Read the model definition and answer for the solid it produces. Units are mm, in the model's axes. A direction names the side the tool comes from. Coordinates: 2 decimals unless noted, no trailing zeros. Order: outer loops, then holes, each group sorted by start corner. A loop starts at its lowest first (then second) coordinate and runs counter-clockwise, first axis right, second up. Notation, with made-up numbers: (53.25, -6) - (101.25, -6) arc R14 cw to (101.25, 16) - close; hole circle Ø2 at (27.5, 9). An arc over 180 degrees is marked (long way). Use one line per item in the form item = value. Start each with the question number.
Autodesk Inventor part; units mm, degrees
ref_plane "YZ Plane" through (0, 0, 0) normal (1, 0, 0) x (0, 1, 0)
ref_plane "XZ Plane" through (0, 0, 0) normal (0, 1, 0) x (-1, 0, 0)
ref_plane "XY Plane" through (0, 0, 0) normal (0, 0, 1) x (1, 0, 0)
sketch "Sketch1" plane through (0, 0, 0) normal (0, 0, 1) x (1, 0, 0)
  circle A0 centre (0, 0) radius 38.1824
extrude "Extrusion1" add sketch "Sketch1" along normal blind 50.8
sketch "Sketch2" plane through (0, 0, 0) normal (0, 0, -1) x (-1, 0, 0)
  line L0 (-10.125, -10.125) -> (10.125, -10.125)
  line L1 (-10.125, 10.125) -> (-10.125, -10.125)
  line L2 (10.125, 10.125) -> (-10.125, 10.125)
  line L3 (10.125, -10.125) -> (10.125, 10.125)
  circle A0 centre (0, 0) radius 25.4
  circle A1 centre (0, 0) radius 25.5
  dimension "d22" = 51
  dimension "d23" = 50.8
extrude "Extrusion2" cut sketch "Sketch2" against normal blind 5 contours L1 L2 L3 L0 | A0 | A1
sketch "Sketch4" plane through (0, 0, 50.8) normal (0, 0, 1) x (1, 0, 0)
  circle A0 centre (0, 0) radius 25.5
  circle A1 centre (0, 0) radius 25.5
extrude "Extrusion4" cut sketch "Sketch4" against normal blind 44.45
ref_plane "Work Plane1" through (0, 10, -2.54) normal (1, 0, 0) x (0, -1, 0)
sketch "Sketch5" plane through (0, 10, -2.54) normal (1, 0, 0) x (0, -1, 0)
  line L0 (-28.1824, -53.34) -> (48.1824, -53.34)
  ellipse E0 centre (10, -53.34) end of major axis (28.5443, -53.34) minor radius 32.3873 (28.5443, -53.34) -> (-8.5443, -53.34) ccw
  point P0 (10, -2.54)
extrude "Extrusion5" cut sketch "Sketch5" along normal through all both and the other way through all
sketch "Sketch6" plane through (0, 10, -2.54) normal (1, 0, 0) x (0, -1, 0)
  point P0 (10, -2.54)
sketch "Sketch7" plane through (0, 0, 6.35) normal (0, 0, 1) x (1, 0, 0)
  circle A0 centre (0, 0) radius 3.975
  circle A1 centre (0, 0) radius 4.1
  dimension "d12" = 8.2
extrude "Extrusion6" cut sketch "Sketch7" against normal blind 10 contours A0 | A1
sketch "Sketch8" plane through (0, 0, 0) normal (0, 0, -1) x (-1, 0, 0)
  circle A0 centre (0, 0) radius 25.4
  line L0 (-17.5031, 18.5443) -> (-33.3767, 18.5443)
  line L1 (-33.3767, -18.5443) -> (-17.5031, -18.5443)
  line L2 (17.5031, -18.5443) -> (33.3767, -18.5443)
  line L3 (33.3767, 18.5443) -> (17.5031, 18.5443)
  circle A1 centre (0, 31.8008) radius 3.4055
  circle A2 centre (-15.9004, 27.5403) radius 3.4055
  circle A3 centre (-27.5403, 15.9004) radius 3.4055
  circle A4 centre (-31.8008, 0) radius 3.4055
  circle A5 centre (-27.5403, -15.9004) radius 3.4055
  circle A6 centre (-15.9004, -27.5403) radius 3.4055
  circle A7 centre (0, -31.8008) radius 3.4055
  circle A8 centre (15.9004, -27.5403) radius 3.4055
  circle A9 centre (27.5403, -15.9004) radius 3.4055
  circle A10 centre (31.8008, 0) radius 3.4055
  circle A11 centre (27.5403, 15.9004) radius 3.4055
  circle A12 centre (15.9004, 27.5403) radius 3.4055
  dimension "d15" = 6.811
  dimension "d18" = 360
sketch "Sketch9" plane through (0, 0, 0) normal (0, 0, -1) x (-1, 0, 0)
  circle A0 centre (0, 31.8008) radius 3.4055
  circle A1 centre (15.9004, 27.5403) radius 3.4055
  circle A2 centre (-15.9004, 27.5403) radius 3.4055
  circle A3 centre (-15.9004, -27.5403) radius 3.4055
  circle A4 centre (0, -31.8008) radius 3.4055
  circle A5 centre (15.9004, -27.5403) radius 3.4055
  circle A6 centre (0, 31.8008) radius 3.4055
  circle A7 centre (15.9004, 27.5403) radius 3.4055
  circle A8 centre (-15.9004, 27.5403) radius 3.4055
  circle A9 centre (-15.9004, -27.5403) radius 3.4055
  circle A10 centre (0, -31.8008) radius 3.4055
  circle A11 centre (15.9004, -27.5403) radius 3.4055
  point P0 (0, 0)
extrude "Extrusion7" cut sketch "Sketch8" against normal blind 48 contours A1 | A2 | A6 | A7 | A8 | A12
properties part number "Launchpad"
Q1. A cutting plane is placed at A-A (x = 0). Give the vertices of the cut face in (y, z).
Q2. A cutting plane is placed at C-C (y = -23). Give the vertices of the cut face in (x, z).
Q3. For a pull along X with two mould halves and no side action, classify faces 1 (the cylindrical face through (-30.3, 23.233, 25.044)), 2 (the flat face through (0, 29, 50.8)), 3 (the flat face through (16, -27, 48)), 4 (the cylindrical face through (5.5, -24.9, 2.5)) as +X half, -X half, draft (parallel to the pull), parting line (faces both ways), or undercut.
Q4. A cutting plane is placed at B-B (z = 29.5). Give the number of separate pieces and of enclosed holes in the cut face, then the cut area to 3 significant figures.
Q5. Given P1, Ø4, axis at x = 15.9, y = 27.54, coming from the -Z side; P2, Ø8, axis at x = 3.5, z = 35.5, coming from the +Y side; P3, Ø1, axis at x = -22, z = 45, coming from the -Y side; P4, Ø5, axis at x = 0, y = 0, coming from the -Z side, each flat-ended and moving along its own axis, determine where each tip first touches the part or whether it passes through.
Q6. Which of the six approach directions +Z, -Z, +X, -X, +Y, -Y give full straight-line access (tool end or side, diameter ignored) to faces 5 (the flat face through (25, -8, 0)), 6 (the cylindrical face through (0.443, 35.177, 23.664)), 7 (the cylindrical face through (13.71, 21.5, 23.95))?
Q7. A cutting plane is placed at D-D (z = 9). Give the vertices of the cut face in (x, y), then the cut area to 3 significant figures.
Q8. Consider probe 1 along Y at (x, z) = (0, 5.3); probe 2 along Y at (x, z) = (0, 29); probe 3 along X at (y, z) = (27.5, 16.5). Determine where each line is inside the solid, lowest interval first.
Result sheet:
q1.outline = (-38.18, 0) - (-35.21, 0) - (-35.21, 48) - (-28.4, 48) - (-28.4, 0) - (-25.5, 0) - (-25.5, 5) - (-4.1, 5) - (-4.1, 6.35) - (-25.5, 6.35) - (-25.5, 50.8) - (-38.18, 50.8) - close; (4.1, 5) - (25.5, 5) - (25.5, 0) - (28.4, 0) - (28.4, 48) - (35.21, 48) - (35.21, 0) - (38.18, 0) - (38.18, 50.8) - (25.5, 50.8) - (25.5, 6.35) - (4.1, 6.35) - close
q2.outline = (-30.48, 0) - (-11.01, 0) - (-11.01, 5) - (11.01, 5) - (11.01, 0) - (30.48, 0) - (30.48, 50.8) - (11.01, 50.8) - (11.01, 6.35) - (-11.01, 6.35) - (-11.01, 50.8) - (-30.48, 50.8) - close
q3.face_1 = parting line
q3.face_2 = draft
q3.face_3 = undercut
q3.face_4 = undercut
q4.separate_pieces = 2
q4.enclosed_holes = 6
q4.area = 1,580 mm^2
q5.P1 = 48
q5.P2 = 38.18
q5.P3 = -31.55
q5.P4 = through
q6.face_5 = -Z, +X, -X, +Y, -Y
q6.face_6 = -Z
q6.face_7 = +Z
q7.outline = circle Ø76.36 at (0, 0); hole circle Ø51 at (0, 0); hole circle Ø6.81 at (-15.9, -27.54); hole circle Ø6.81 at (-15.9, 27.54); hole circle Ø6.81 at (0, -31.8); hole circle Ø6.81 at (0, 31.8); hole circle Ø6.81 at (15.9, -27.54); hole circle Ø6.81 at (15.9, 27.54)
q7.area = 2,320 mm^2
q8.probe_1 = -38.18 to -35.21, -28.4 to -4.1, 4.1 to 28.4, 35.21 to 38.18
q8.probe_2 = -38.18 to -35.21, -28.4 to -25.5, 25.5 to 28.4, 35.21 to 38.18
q8.probe_3 = -26.49 to -19.31, -12.5 to 12.5, 19.31 to 26.49
